Model file for the job. Use its own axes, mm. Face numbers are marked on the shaded views. A direction names the side the tool comes from. Coordinates: 2 decimals unless noted, no trailing zeros. Write each loop counter-clockwise with the first axis right and the second up, starting at its lowest first coordinate (ties: lowest second). Pieces come first, ordered by that corner, then holes. Notation, with made-up numbers: M 49.5,-25 L 79.5,-25 A31 cw 79.5,6 Z; hole C -10,44 d7. An arc over 180 degrees is marked long. Answer in a Markdown table with one row per item. Add a question column.
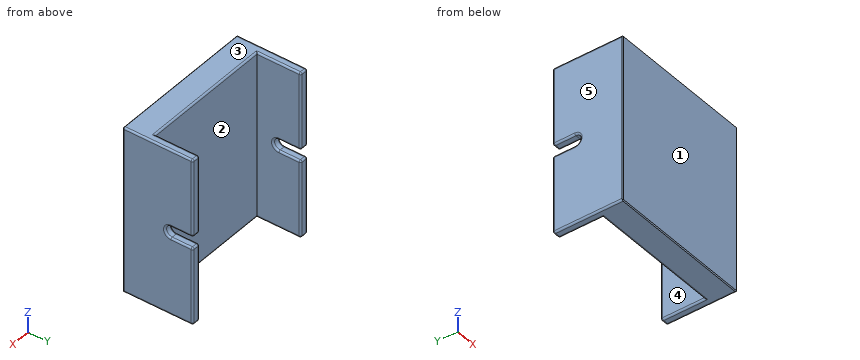
```python
from build123d import *

# Parameters (mm, degrees)
SKETCH2_W           = 85.7504
SKETCH2_H           = 96.2
BOSS_EXTRUDE1_DEPTH = 15
SKETCH2_3_W         = 4.7752
SKETCH2_3_H         = 86.2
SKETCH2_3_H_2       = 10
BOSS_EXTRUDE2_DEPTH = 25.4
CUT_EXTRUDE1_DEPTH  = 86.7504
CHAMFER1_SIZE       = 0.5
FILLET2_R           = 1


with BuildPart() as part:
    # Sketch2 → Boss-Extrude1 (new body)
    with BuildSketch(Plane(origin=(0, 34, 0), x_dir=(-1, 0, 0), z_dir=(0, -1, 0))):
        with Locations((-150, -48.1)):
            Rectangle(SKETCH2_W, SKETCH2_H)
    extrude(amount=BOSS_EXTRUDE1_DEPTH)

    # Sketch2_3 → Boss-Extrude2 (add)
    with BuildSketch(Plane(origin=(0, 34, 0), x_dir=(-1, 0, 0), z_dir=(0, -1, 0))):
        with Locations((-109.5124, -53.1)):
            Rectangle(SKETCH2_3_W, SKETCH2_3_H)
        with Locations((-109.5124, -5)):
            Rectangle(SKETCH2_3_W, SKETCH2_3_H_2)
        with Locations((-190.4876, -53.1)):
            Rectangle(SKETCH2_3_W, SKETCH2_3_H)
        with Locations((-190.4876, -5)):
            Rectangle(SKETCH2_3_W, SKETCH2_3_H_2)
    extrude(amount=-BOSS_EXTRUDE2_DEPTH)

    # Sketch3 → Cut-Extrude1 (cut, through all)
    with BuildSketch(Plane(origin=(192.8752, 0, 0), x_dir=(0, 0, -1), z_dir=(1, 0, 0))):
        with BuildLine():
            Line((-51.3639, 46.7), (-51.3639, 59.4))
            Line((-51.3639, 59.4), (-44.8361, 59.4))
            Line((-44.8361, 59.4), (-44.8361, 46.7))
            ThreePointArc((-44.8361, 46.7), (-48.1, 43.4361), (-51.3639, 46.7))
        make_face()
    extrude(amount=-CUT_EXTRUDE1_DEPTH, mode=Mode.SUBTRACT)

    # Chamfer1
    chamfer1_edges = [part.edges().sort_by_distance(p)[0] for p in [
        (192.8752, 19, 48.1),
        (150, 19, 0),
        (107.1248, 19, 48.1),
        (150, 19, 96.2),
    ]]
    chamfer(chamfer1_edges, length=CHAMFER1_SIZE)

    # Fillet2
    fillet2_edges = [part.edges().sort_by_distance(p)[0] for p in [
        (150, 34, 96.2),
        (150, 34, 0),
        (111.9, 46.7, 96.2),
        (109.5124, 59.4, 0),
        (111.9, 46.7, 0),
        (107.1248, 59.4, 22.41805),
        (109.5124, 59.4, 96.2),
        (111.9, 59.4, 73.78195),
        (188.1, 59.4, 73.78195),
        (188.1, 46.7, 0),
        (188.1, 46.7, 96.2),
        (192.8752, 59.4, 22.41805),
        (190.4876, 59.4, 0),
        (190.4876, 59.4, 96.2),
        (188.1, 59.4, 22.41805),
        (192.8752, 59.4, 73.78195),
        (190.4876, 59.4, 51.3639),
        (190.4876, 59.4, 44.8361),
        (188.1, 43.4361, 48.1),
        (107.1248, 59.4, 73.78195),
        (111.9, 59.4, 22.41805),
        (111.9, 43.4361, 48.1),
        (107.1248, 43.4361, 48.1),
        (109.5124, 59.4, 51.3639),
        (109.5124, 59.4, 44.8361),
        (111.9, 53.05, 44.8361),
        (107.1248, 53.05, 44.8361),
        (188.1, 53.05, 44.8361),
        (111.9, 53.05, 51.3639),
        (107.1248, 53.05, 51.3639),
        (188.1, 53.05, 51.3639),
        (192.8752, 53.05, 44.8361),
        (192.8752, 53.05, 51.3639),
        (192.8752, 43.4361, 48.1),
        (107.1248, 39.45, 96.2),
        (192.8752, 39.45, 96.2),
        (192.8752, 39.45, 0),
        (107.1248, 39.45, 0),
    ]]
    fillet(fillet2_edges, radius=FILLET2_R)


solid = part.part
```
1) Slice it at C-C (x = 180). Give the cut face in (y, z).
2) Which spindle directions (+Z, -Z, +X, -X, +Y, -Y) get a long thin tool onto all of the face, cutting with end or side? Do the marked faces 1 and 2. Say none if no direction does.
3) Flat gauge pins, fed straight in: pin 1 Ø1.5 at (y, z) = (45, 46) entering from -X; pin 2 Ø3 at (x, z) = (178, 70) entering from +Y; pin 3 Ø4 at (y, z) = (44, 50) entering from -X. Where does each tip first touch, or does it go through?
4) Slice it at B-B (z = 48.1). Give the cut face in (x, y).
5) Slice it at A-A (y = 48.5). Count the separate pieces of the cut face and the enclosed holes in it, then the cut area to 3 significant figures.
6) Drill centre lines: probe 1 along X at (y, z) = (34.5, 61); probe 2 along Y at (x, z) = (156, 54); probe 3 along Z at (x, y) = (189, 47). Where is each one in solid material? Low to high.
7) Slice it at D-D (z = 19). Give the cut face in (x, y), then the cut area to 3 significant figures.
8) Two-plate mould, pull along X, no slides. Class the marked faces 3, 4 and 5: released by +X, released by -X, zero draft, split by the parting line, or undercut.
Ans:
| question | item | result |
|---|---|---|
| 1 | outline | M 19,0.5 L 19.5,0 L 33,0 A1 ccw 34,1 L 34,95.2 A1 ccw 33,96.2 L 19.5,96.2 L 19,95.7 Z |
| 2 | face 1 | +Z, -Z, +X, -X, -Y |
| 2 | face 2 | +Z, -Z, +Y |
| 3 | pin 1 | stops at x = 107.54 |
| 3 | pin 2 | stops at y = 34 |
| 3 | pin 3 | stops at x = 107.12 |
| 4 | outline | M 107.12,19.5 L 107.62,19 L 192.38,19 L 192.88,19.5 L 192.88,42.44 A1 ccw 191.88,43.44 L 189.1,43.44 A1 ccw 188.1,42.44 L 188.1,34 L 111.9,34 L 111.9,42.44 A1 ccw 110.9,43.44 L 108.12,43.44 A1 ccw 107.12,42.44 Z |
| 5 | separate pieces | 4 |
| 5 | enclosed holes | 0 |
| 5 | area | 853 mm2 |
| 6 | probe 1 | x = 107.12 to 111.9, 188.1 to 192.88 |
| 6 | probe 2 | y = 19 to 34 |
| 6 | probe 3 | z = 0.01 to 44.83, 51.37 to 96.19 |
| 7 | outline | M 107.12,19.5 L 107.62,19 L 192.38,19 L 192.88,19.5 L 192.88,58.4 A1 ccw 191.88,59.4 L 189.1,59.4 A1 ccw 188.1,58.4 L 188.1,34 L 111.9,34 L 111.9,58.4 A1 ccw 110.9,59.4 L 108.12,59.4 A1 ccw 107.12,58.4 Z |
| 7 | area | 1,530 mm2 |
| 8 | face 3 | zero draft |
| 8 | face 4 | undercut |
| 8 | face 5 | released by -X |
